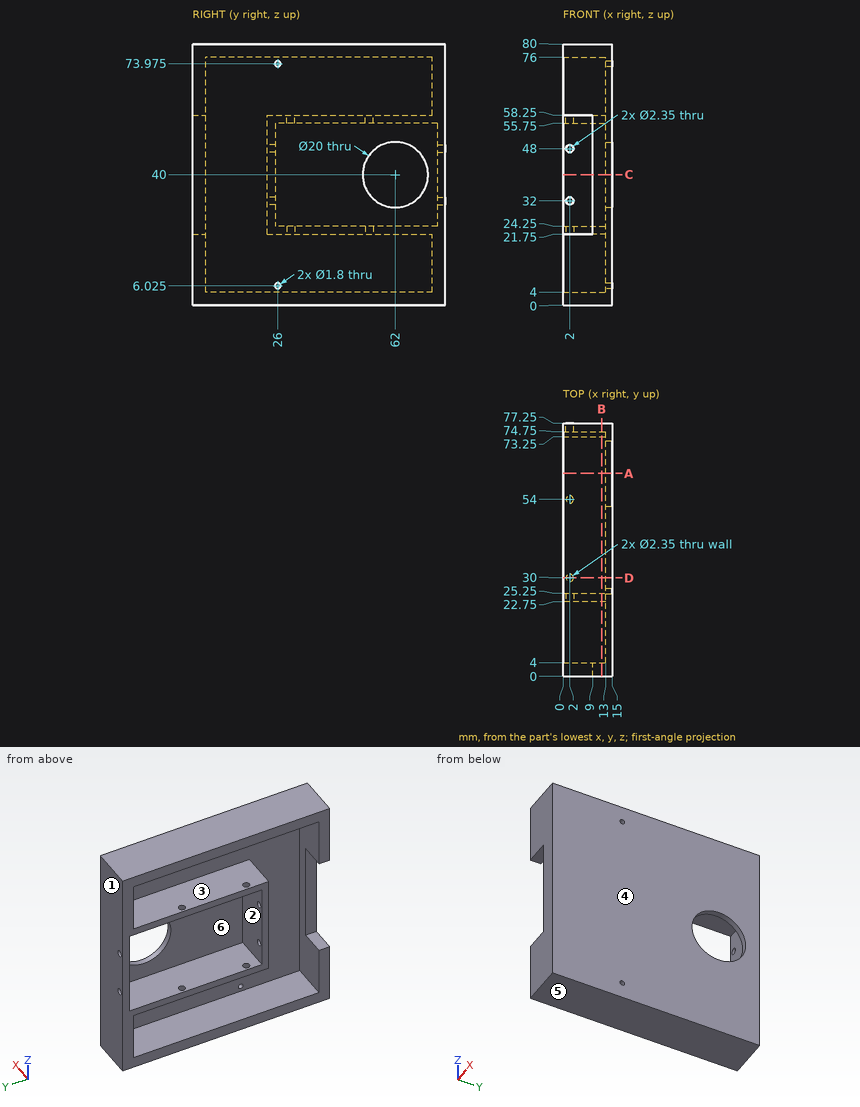
Geometry: see drawing. Coordinates: mm, zero at the bounding-box minimum. A direction names the side the tool comes from. Coordinates: 2 decimals unless noted, no trailing zeros. Write each loop counter-clockwise with the first axis right and the second up, starting at its lowest first coordinate (ties: lowest second). Pieces come first, ordered by that corner, then holes. Notation, with made-up numbers: M 17.25,45.5 L 61.25,45.5 A10 cw 61.25,51.5 Z; hole C 40,57.25 d11. An arc over 180 degrees is marked long. Answer as a JSON object with one key per item and string values.
1. Cut plane C-C on z = 40. Output: boundary loops of the cut face in (x, y), plus the area to 4 significant figures.
Evaluation:
{"outline": "M 0,22.75 L 13,22.75 L 13,4 L 9,4 L 9,0 L 15,0 L 15,52 L 13,52 L 13,25.25 L 0,25.25 Z; M 0,74.75 L 13,74.75 L 13,72 L 15,72 L 15,77.25 L 0,77.25 Z", "area": "195.5 mm^2"}
2. Contact query for flat-ended pins moving along their axis: P1, Ø5, axis at y = 58, z = 9, coming from the -X side; P2, Ø1.2, axis at y = 1, z = 42, coming from the -X side. Output: stop coordinate, or through.
Evaluation:
{"P1": "x = 13", "P2": "x = 9"}
3. Access query for the marked faces 1 and 2. Directions: +Z, -Z, +X, -X, +Y, -Y. A direction counts if a zero-diameter tool reaches every point of the face in a straight line with its end or side. Return the directions, or none.
Evaluation:
{"face 1": "+Z, -Z, +X, -X, +Y", "face 2": "-X"}
4. Draft query along Z for the marked faces 3, 4, 5 and 6. Return one class per face: released by +Z, released by -Z, zero draft, split by the parting line, or undercut.
Evaluation:
{"face 3": "undercut", "face 4": "zero draft", "face 5": "released by -Z", "face 6": "undercut"}
5. Cut plane A-A on y = 62. Output: boundary loops of the cut face in (x, z), plus the area to 3 significant figures.
Evaluation:
{"outline": "M 0,0 L 15,0 L 15,30 L 13,30 L 13,24.25 L 0,24.25 L 0,21.75 L 13,21.75 L 13,4 L 0,4 Z; M 0,55.75 L 13,55.75 L 13,50 L 15,50 L 15,80 L 0,80 L 0,76 L 13,76 L 13,58.25 L 0,58.25 Z", "area": "289 mm^2"}
6. Cut plane D-D on y = 30. Output: boundary loops of the cut face in (x, z) (3 decimals).
Evaluation:
{"outline": "M 0,0 L 15,0 L 15,80 L 0,80 L 0,76 L 13,76 L 13,58.25 L 3.175,58.25 L 3.175,55.75 L 13,55.75 L 13,24.25 L 3.175,24.25 L 3.175,21.75 L 13,21.75 L 13,4 L 0,4 Z; M 0,21.75 L 0.825,21.75 L 0.825,24.25 L 0,24.25 Z; M 0,55.75 L 0.825,55.75 L 0.825,58.25 L 0,58.25 Z"}
7. Ray query, L1, parallel to Z at x = 1, y = 42; L2, parallel to Y at x = 2, z = 56.3 (3 decimals); L3, parallel to Z at x = 2, y = 24.4 (3 decimals). Return the intervals inside material, ascending.
Evaluation:
{"L1": "0 to 4, 21.75 to 24.25, 55.75 to 58.25, 76 to 80", "L2": "22.75 to 28.825, 31.175 to 52.825, 55.175 to 77.25", "L3": "0 to 4, 21.75 to 30.825, 33.175 to 46.825, 49.175 to 58.25, 76 to 80"}
8. Cut plane B-B on x = 11.75. Output: boundary loops of the cut face in (y, z).
Evaluation:
{"outline": "M 0,0 L 77.25,0 L 77.25,80 L 0,80 Z; hole M 4,4 L 73.25,4 L 73.25,21.75 L 22.75,21.75 L 22.75,58.25 L 73.25,58.25 L 73.25,76 L 4,76 Z; hole M 25.25,24.25 L 74.75,24.25 L 74.75,55.75 L 25.25,55.75 Z"}
